Could you check a few things on this drawing? It's one solid part, dimensions in mm from its lowest x, y, z. A direction names the side the tool comes from. Give positions to 0.01 mm unless a question says otherwise; leave off trailing zeros. Loops run counter-clockwise (first coordinate to the right, second up) from the corner with the lowest first, then second, coordinate; pieces in that order, holes last. Notation, with made-up numbers: (7, 56) - (24, 56) arc R24 ccw to (24, 81) - close; hole circle Ø3 at (-17, 38). An arc over 180 degrees is marked (long way). Use CSV: the item, a comma, the result in double quotes.
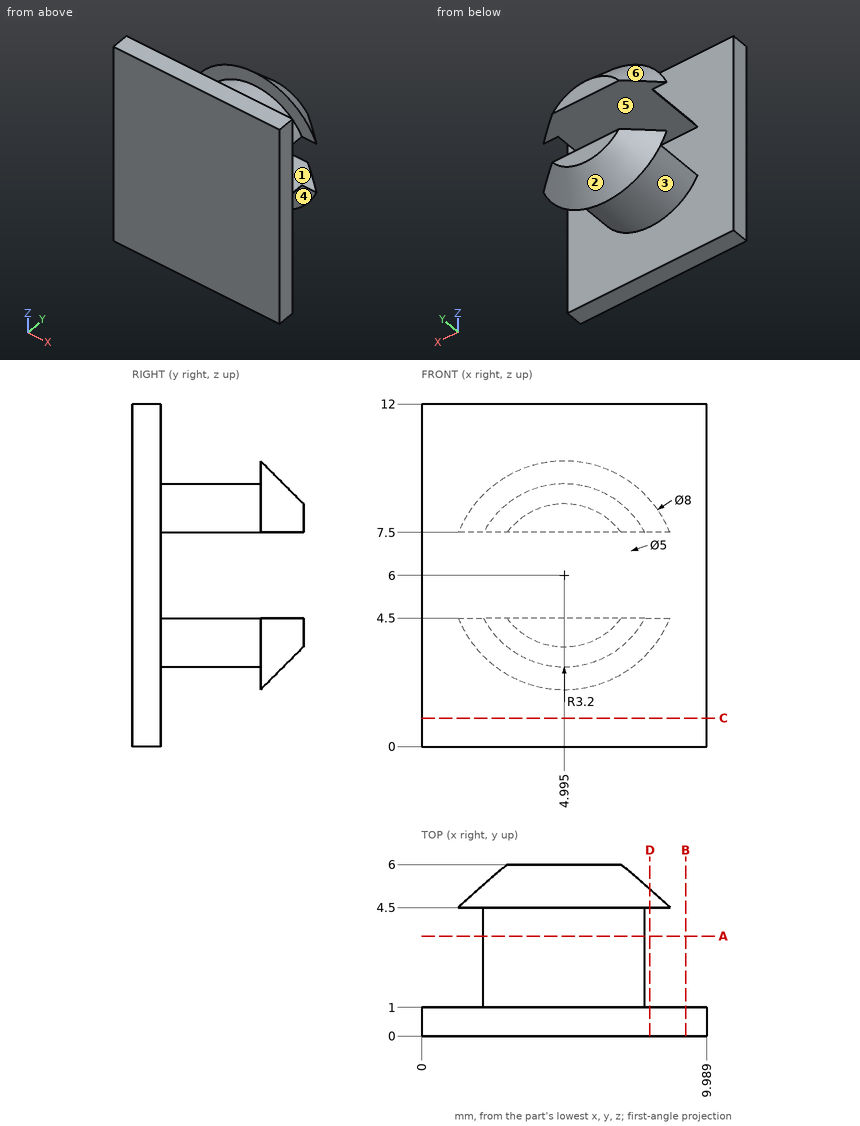
1) Which directions (+Z, -Z, +X, -X, +Y, -Y) give clear straight access to the entire face, cutting with the end or side of a thin tool? Please do the marked faces 1, 2 and 3.
Answer below:
face 1,"+X, -X, +Y"
face 2,"-Z, +Y"
face 3,"-Z"
2) Suppose I cut it at D-D (x = 8). State how many separate pieces and enclosed holes the cut face has.
Answer below:
separate pieces,"3"
enclosed holes,"0"
3) I need wall thicknesses on line 1 along Z through (x, y) = (3, 3) (1 decimal); line 2 along Y through (x, z) = (2.75, 11); line 3 along Z through (x, y) = (3.75, 2.25). Which ranges of each line are inside material? Lowest first, please.
Answer below:
line 1,"z = 3.5 to 4.5, 7.5 to 8.5"
line 2,"y = 0 to 1"
line 3,"z = 3.05 to 4.5, 7.5 to 8.95"
4) I'm going to push flat-ended pins straight in: P1, Ø1.5, axis at x = 7, y = 2.5, coming from the -Z side; P2, Ø2, axis at x = 3.5, z = 8.5, coming from the -Y side; P3, Ø1.5, axis at x = 3.5, y = 4, coming from the +Z side. Where does each tip first touch, or does it pass through?
Answer below:
P1,"stops at z = 3.06"
P2,"stops at y = 0"
P3,"stops at z = 9.89"
5) Suppose I cut it at C-C (z = 1). Please give me the cut outline in (x, y).
Answer below:
outline,"(0, 0) - (9.99, 0) - (9.99, 1) - (0, 1) - close"
6) We'd pull the mould along Y, two halves only. Please class the marked faces 4, 5 and 6: +Y half, -Y half, draft (parallel to the pull), parting line (faces both ways), or undercut.
Answer below:
face 4,"undercut"
face 5,"draft"
face 6,"+Y half"
7) Suppose I cut it at A-A (y = 3.5). Please give me the cut outline in (x, z) (1 decimal), plus the area to 3 significant figures.
Answer below:
outline,"(2.2, 4.5) arc R3.2 ccw to (7.8, 4.5) - close; (2.2, 7.5) - (7.8, 7.5) arc R3.2 ccw to start"
area,"13.7 mm2"
8) Suppose I cut it at B-B (x = 9.25). Please give me the cut outline in (y, z), plus the area to 3 significant figures.
Answer below:
outline,"(0, 0) - (1, 0) - (1, 12) - (0, 12) - close"
area,"12.0 mm2"
